Here's how the part is built. I have some questions about the finished solid (model axes, mm). Face numbers are marked on the shaded views. Round coordinates to 2 decimals unless told otherwise and drop trailing zeros. Write each loop counter-clockwise with the first axis right and the second up, starting at its lowest first coordinate (ties: lowest second). Pieces come first, ordered by that corner, then holes. Notation, with made-up numbers: (36, 25.5) -> (59, 25.5) arc R29 ccw to (59, 54.5) -> close; hole circle Ø1 at (-2, 23). An arc over 180 degrees is marked (long way). Answer in a Markdown table with one row per item. Add a question column.
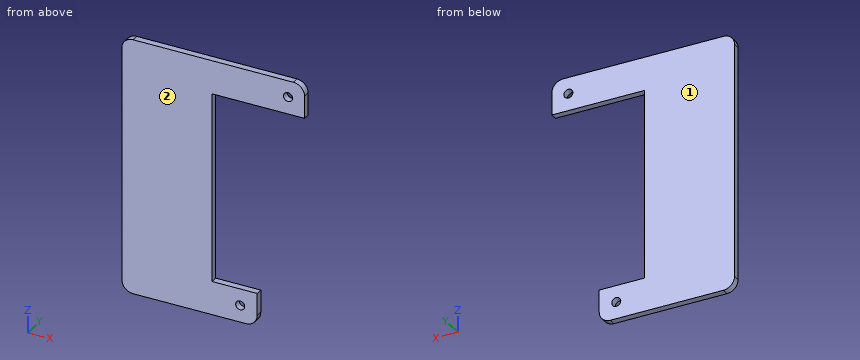
from build123d import *

# Parameters (mm, degrees)
F0_R     = 2
F1_DEPTH = 3
F2_R     = 5


# Not quite as in the source:
# - a feature names something its author has since deleted; it is built from what else it names


with BuildPart() as f1:
    # F0 (on Front) → F1 (new body)
    with BuildSketch(Plane.XZ):
        Polygon((-81, 51.5256257355), (-81, -63.4743742645), (-21, -63.4743742645), (-21, -48.4743742645), (-41, -48.4743742645), (-41, -15.9743742645), (-41, 4.0256257355), (-41, 36.5256257355), (0, 36.5256257355), (0, 51.5256257355), align=None)
        with Locations((-28.5549983382, -55.90621382)):
            Circle(F0_R, mode=Mode.SUBTRACT)
        with Locations((-7.3309438303, 44.1784150898)):
            Circle(F0_R, mode=Mode.SUBTRACT)
    extrude(amount=F1_DEPTH)

    # F2
    f2_edges = [f1.edges().sort_by_distance(p)[0] for p in [
        (-81, -1.5, 51.525626),
        (-81, -1.5, -63.474374),
        (0, -1.5, 51.525626),
        (-21, -1.5, -63.474374),
    ]]
    fillet(f2_edges, radius=F2_R)


solid = f1.part
Item 1: If we mould it in two halves opening along Y, with no side actions, what happens to the marked faces 1 and 2? For each: pulls with the +Y half, pulls with the -Y half, needs draft (parallel to the pull), parting line crosses it, or undercut.
Item 2: I need wall thicknesses on line 1 along Z through (x, y) = (-28, -1.8); line 2 along X through (y, z) = (-2.7, 19); line 3 along Z through (x, y) = (-14, -1.2). Which ranges of each line are inside material? Lowest first, please. Write a range as from..to.
Item 3: If we section it at A-A on x = -8: Please give me the cut outline in (y, z), then the cut area to 3 significant figures.
Item 4: If we section it at C-C on z = 31.5: Please give me the cut outline in (x, y).
Item 5: If we section it at B-B on y = -1.75: Please give me the cut outline in (x, z) (3 decimals).
Results list:
| question | item | result |
|---|---|---|
| 1 | face 1 | pulls with the +Y half |
| 1 | face 2 | pulls with the -Y half |
| 2 | line 1 | -63.47..-57.83, -53.98..-48.47, 36.53..51.53 |
| 2 | line 2 | -81..-41 |
| 2 | line 3 | 36.53..51.53 |
| 3 | outline | (-3, 36.53) -> (0, 36.53) -> (0, 42.29) -> (-3, 42.29) -> close; (-3, 46.06) -> (0, 46.06) -> (0, 51.53) -> (-3, 51.53) -> close |
| 3 | area | 33.7 mm² |
| 4 | outline | (-81, -3) -> (-41, -3) -> (-41, 0) -> (-81, 0) -> close |
| 5 | outline | (-81, -58.474) arc R5 ccw to (-76, -63.474) -> (-26, -63.474) arc R5 ccw to (-21, -58.474) -> (-21, -48.474) -> (-41, -48.474) -> (-41, 36.526) -> (0, 36.526) -> (0, 46.526) arc R5 ccw to (-5, 51.526) -> (-76, 51.526) arc R5 ccw to (-81, 46.526) -> close; hole circle Ø4 at (-28.555, -55.906); hole circle Ø4 at (-7.331, 44.178) |
